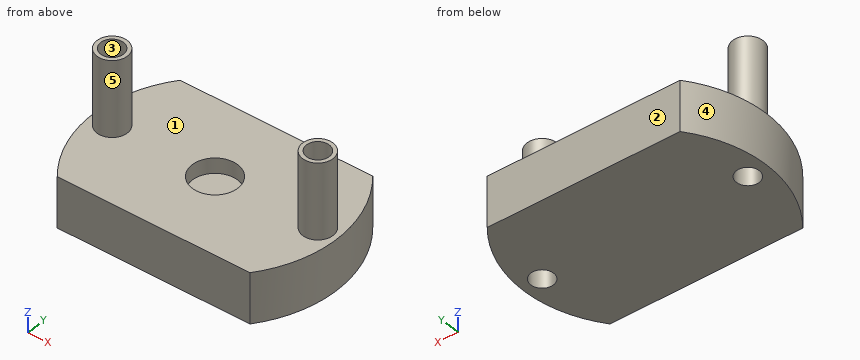
Autodesk Fusion 360 part; units mm, degrees
sketch "Esquisse1" plane through (0, 0, 0) normal (0, 0, 1) x (1, 0, 0)
  circle A0 centre (0, 0) radius 24
  dimension "d1" = 48
extrude "Extrusion1" add sketch "Esquisse1" along normal blind 10
sketch "Esquisse2" plane through (0, 0, 10) normal (0, 0, 1) x (-1, 0, 0)
  circle A0 centre (0, 0) radius 24
  circle A1 centre (0, 0) radius 4.5
  dimension "d4" = 9
extrude "Extrusion2" cut sketch "Esquisse2" against normal blind 3 contours A1
sketch "Esquisse3" plane through (0, 0, 10) normal (0, 0, 1) x (-1, 0, 0)
  circle A0 centre (0, 0) radius 4.5
  circle A1 centre (0, 0) radius 24
  circle A2 centre (20, 0) radius 3
  dimension "d7" = 20
  dimension "d17" = 6
extrude "Extrusion3" add sketch "Esquisse3" along normal blind 15 contours A2
mirror "Symétrie miroir1" about plane through (0, 0, 0) normal (1, 0, 0) of "Extrusion3"
sketch "Esquisse4" plane through (0, 0, 25) normal (0, 0, 1) x (-1, 0, 0)
  circle A0 centre (20, 0) radius 3
  circle A1 centre (20, 0) radius 2.25
  dimension "d12" = 4.5
extrude "Extrusion4" cut sketch "Esquisse4" against normal blind 36 contours A1
mirror "Symétrie miroir2" about plane through (0, 0, 0) normal (1, 0, 0) of "Extrusion4"
sketch "Esquisse5" plane through (0, 0, 10) normal (0, 0, 1) x (-1, 0, 0)
  circle A0 centre (-20, 0) radius 3
  circle A1 centre (20, 0) radius 3
  circle A2 centre (0, 0) radius 4.5
  circle A3 centre (0, 0) radius 24
sketch "Esquisse6" plane through (0, 0, 10) normal (0, 0, 1) x (-1, 0, 0)
  line L0 (29.6799, -30) -> (-29.6799, -30)
  line L1 (-29.6799, -30) -> (-29.6799, -15)
  line L2 (-29.6799, -15) -> (29.6799, -15)
  line L3 (29.6799, -15) -> (29.6799, -30)
  line L4 (0, -1.75) -> (0, -22.5)
  line L5 (-20, 0) -> (-2.5, 0)
  dimension "d18" = 15
  dimension "d19" = 15
extrude "Extrusion5" cut sketch "Esquisse6" against normal blind 25
mirror "Symétrie miroir3" about plane through (0, 0, 0) normal (0, 1, 0) of "Extrusion5"
Check sheet for the modelled part. Datum: model origin and axes. Units: mm. Face numbers are marked on the shaded views. A direction names the side the tool comes from. Round coordinates to 2 decimals unless told otherwise and drop trailing zeros. Order: outer loops, then holes, each group sorted by start corner. A loop starts at its lowest first (then second) coordinate and runs counter-clockwise, first axis right, second up.
(1) Cross-section at B-B, the plane x = 0. Enter the section's corners in (y, z), and give its area (3 significant figures).
(2) Draft check along Y on the marked faces 1, 2 and 3. Enter one of: pulls with the +Y half, pulls with the -Y half, needs draft (parallel to the pull), parting line crosses it, or undercut.
(3) Go/stop test with flat-tipped pins: P1, Ø6, axis at y = -11.5, z = 7, coming from the +X side; P2, Ø11.5, axis at x = 0, y = 0, coming from the +Z side; P3, Ø4.5, axis at x = 0, y = 2, coming from the +Z side. Record where each tip stops, or that it passes through.
(4) Scan lines: probe 1 along X at (y, z) = (0, 13); probe 2 along X at (y, z) = (0, 9.1); probe 3 along Y at (x, z) = (-20, 18.75). Record each from-to range of solid material in increasing order.
(5) Access from +Z, -Z, +X, -X, +Y, -Y to the whole of each face (thin tool, end or side, straight path). Record for the marked faces 4 and 5.
(6) Cross-section at A-A, the plane y = 0. Enter the section's corners in (x, z).
(7) Cross-section at C-C, the plane z = 3. Enter the section's corners in (x, y) (3 decimals).
(8) Cross-section at D-D, the plane x = 20. Enter the section's corners in (y, z).
Check sheet entries:
1. outline: (-15, 0) - (15, 0) - (15, 10) - (4.5, 10) - (4.5, 7) - (-4.5, 7) - (-4.5, 10) - (-15, 10) - close
1. area: 273 mm2
2. face 1: needs draft
2. face 2: pulls with the +Y half
2. face 3: undercut
3. P1: stops at x = 22.44
3. P2: stops at z = 10
3. P3: stops at z = 7
4. probe 1: x = -23 to -22.25, -17.75 to -17, 17 to 17.75, 22.25 to 23
4. probe 2: x = -24 to -22.25, -17.75 to -4.5, 4.5 to 17.75, 22.25 to 24
4. probe 3: y = -3 to -2.25, 2.25 to 3
5. face 4: +Z, -Z, -X
5. face 5: +Z
6. outline: (-24, 0) - (-22.25, 0) - (-22.25, 25) - (-23, 25) - (-23, 10) - (-24, 10) - close; (-17.75, 0) - (17.75, 0) - (17.75, 25) - (17, 25) - (17, 10) - (4.5, 10) - (4.5, 7) - (-4.5, 7) - (-4.5, 10) - (-17, 10) - (-17, 25) - (-17.75, 25) - close; (22.25, 0) - (24, 0) - (24, 10) - (23, 10) - (23, 25) - (22.25, 25) - close
7. outline: (-18.735, -15) - (18.735, -15) arc R24 ccw to (18.735, 15) - (-18.735, 15) arc R24 ccw to start; hole circle Ø4.5 at (-20, 0); hole circle Ø4.5 at (20, 0)
8. outline: (-13.27, 0) - (-2.25, 0) - (-2.25, 25) - (-3, 25) - (-3, 10) - (-13.27, 10) - close; (2.25, 0) - (13.27, 0) - (13.27, 10) - (3, 10) - (3, 25) - (2.25, 25) - close
